from build123d import *

# Parameters (mm, degrees)
F2_R     = 2.2337294629
F3_DEPTH = 94.1962972283
F4_R     = 5.08


with BuildPart() as f1:
    # F0 (on Right) → F1 (revolve)
    with BuildSketch(Plane.YZ):
        Polygon((87.180994451, 6.4897), (100.203, 6.4897), (100.203, 6.0571772046), (181.6655695438, 6.0571772046), (181.6655695438, 9.5376558602), (100.203, 9.5376558602), (81.7666972255, 15.7631933689), (0, 15.7631933689), (0, 10.2108), (6.6675017588, 10.2108), (76.3524, 10.2108), align=None)
    revolve(axis=Axis((0, 3.5269334912, 0), (0, 1, 0)))

    # F2
    f2_edges = [f1.edges().sort_by_distance(p)[0] for p in [
        (0, 0, -10.2108),
    ]]
    fillet(f2_edges, radius=F2_R)

    # F3 (add): a face of the model
    f3_faces = [f1.faces().sort_by_distance(p)[0] for p in [
        (0, 181.6655695438, -6.3269428501),
    ]]
    extrude(f3_faces, amount=F3_DEPTH)

    # F4
    f4_edges = [f1.edges().sort_by_distance(p)[0] for p in [
        (0, 81.766697, -15.763193),
        (0, 100.203, -9.537656),
    ]]
    fillet(f4_edges, radius=F4_R)


solid = f1.part
Design review of the part built by this model. Coordinates are the model's own, in mm. A direction names the side the tool comes from. Coordinates: 2 decimals unless noted, no trailing zeros. Order: outer loops, then holes, each group sorted by start corner. A loop starts at its lowest first (then second) coordinate and runs counter-clockwise, first axis right, second up. Notation, with made-up numbers: (77, -28.75) -> (84, -28.75) arc R36 ccw to (84, 7.25) -> close; hole circle Ø3 at (-19.5, 52). An arc over 180 degrees is marked (long way). One line per item, written item: value.
1) We need section B-B, the plane y = 60.5. Give the boundary of the cut face in (x, z).
Output values:
outline: circle Ø31.53 at (0, 0); hole circle Ø20.42 at (0, 0)
2) To check wall thickness, follow probe 1 along X at (y, z) = (25.5, 0); probe 2 along Z at (x, y) = (-7, 15); probe 3 along Z at (x, y) = (5.5, 147.5). State the ranges of each line that lie inside material, in increasing order. Write a range as [from, to].
Output values:
probe 1: x = [-15.76, -10.21], [10.21, 15.76]
probe 2: z = [-14.12, -7.43], [7.43, 14.12]
probe 3: z = [-7.79, -2.54], [2.54, 7.79]
3) Machinability: for faces 4 (the face through (5, 0, 12)), 5 (the face through (-6, 100.203, -2)), 6 (the face through (2.86, 187.23, 9.1)), which of the approach directions +Z, -Z, +X, -X, +Y, -Y give a long, thin tool a straight path to every point of the face, cutting with its end or side? Answer none if there is none.
Output values:
face 4: +Z, -Z, +X, -X, -Y
face 5: -Y
face 6: +Y
4) Draft analysis for pull direction Z (two halves, no side actions). For faces 1 (the face through (-6.22, 275.862, 0.13)), 2 (the face through (4.735, 39.9, 15.035)), 3 (the face through (-6.335, 93.783, -1.407)), state which applies: +Z half, -Z half, draft (parallel to the pull), parting line (faces both ways), or undercut.
Output values:
face 1: draft
face 2: parting line
face 3: undercut
5) Clearance check with flat-ended pins moving along their axes: P1, Ø9.5, axis at x = 0, z = 0, coming from the +Y side; P2, Ø10, axis at y = 56.5, z = 7, coming from the +X side; P3, Ø10, axis at y = 160, z = 12.5, coming from the -X side; P4, Ø6, axis at x = -8, y = 172, coming from the +Z side. State where each tip first meets the part, or that it passes through.
Output values:
P1: passes through
P2: stops at x = 15.64
P3: stops at x = -5.89
P4: stops at z = 8.12
6) We need section A-A, the plane y = 254.5. Give the boundary of the cut face in (x, z).
Output values:
outline: circle Ø19.08 at (0, 0); hole circle Ø12.11 at (0, 0)
